Read the model definition and answer for the solid it produces. Units are mm, in the model's axes. A direction names the side the tool comes from. Round coordinates to 2 decimals unless told otherwise and drop trailing zeros. Order: outer loops, then holes, each group sorted by start corner. A loop starts at its lowest first (then second) coordinate and runs counter-clockwise, first axis right, second up. Notation, with made-up numbers: (46.25, 74) -> (74.25, 74) arc R10 cw to (74.25, 91) -> close; hole circle Ø11 at (-35.75, 83). An arc over 180 degrees is marked (long way). Use a Markdown table: item, result. Add a question column.
1. Section A-A, the plane z = 3.25 is taken. Give the vertices of the cut face in (x, y), then the cut area to 3 significant figures.
2. Section C-C, the plane x = 70 is taken. Give the vertices of the cut face in (y, z).
3. Given pin 1 (2.5 mm diameter, centred on y = -5.5, z = 18, fed in from +X); pin 2 (10 mm diameter, centred on x = 169.5, z = 6.5, fed in from -Y); pin 3 (4 mm diameter, centred on x = 310, z = 10, fed in from -Y); pin 4 (4.5 mm diameter, centred on x = 10, z = 10, fed in from +Y), each flat-ended and moving along its own axis, determine where each tip first touches the part or whether it passes through.
4. Consider L1, parallel to X at y = 13.95, z = 10; L2, parallel to Z at x = 10, y = 13.2; L3, parallel to X at y = 12, z = 12. Determine where each line is inside the solid, lowest interval first. Write a range as [from, to].
5. The mould has two halves that part along Y. Classify faces 1 (the face through (20, -12, 18)), 2 (the face through (10, -33, 18)), 3 (the face through (10, -12, 15)), 4 (the face through (158, 15, 10)): +Y half, -Y half, draft (parallel to the pull), parting line (faces both ways), or undercut.
6. Section B-B, the plane y = -15.8 is taken. Give the vertices of the cut face in (x, z), then the cut area to 4 significant figures.
7. Section D-D, the plane y = -28 is taken. Give the vertices of the cut face in (x, z), then the cut area to 3 significant figures.
8. For faces 5 (the face through (12.32, -17.93, 7.6)), 6 (the face through (9.46, 12.54, 12.44)), 7 (the face through (0, -4, 16)), determine the directions among +Z, -Z, +X, -X, +Y, -Y from which every point of the face is accessible in a straight line to the end or side of a thin tool.
Autodesk Inventor part; units mm, degrees
ref_plane "Plano de trabajo1" through (0, 10, 0) normal (0, 1, 0) x (1, 0, 0)
ref_plane "Plano de trabajo4" through (0, -3, 0) normal (0, -1, 0) x (1, 0, 0)
ref_plane "Plano de trabajo5" through (20, -33, 15) normal (0, 0, -1) x (-1, 0, 0)
ref_plane "Plano de trabajo1" through (0, 10, 0) normal (0, 1, 0) x (1, 0, 0)
sketch "Boceto3" plane through (0, 10, 0) normal (0, 1, 0) x (1, 0, 0)
  line L0 (20, -20) -> (0, -20)
  line L1 (0, 0) -> (20, 0)
  line L2 (0, -20) -> (20, -20)
  line L3 (20, -20) -> (20, 0)
  line L4 (20, 0) -> (0, 0)
  line L5 (0, 0) -> (0, -20)
extrude "Extrusión3" add sketch "Boceto3" along normal blind 5
ref_plane "Plano de trabajo4" through (0, -3, 0) normal (0, -1, 0) x (1, 0, 0)
sketch "Boceto8" plane through (0, -3, 0) normal (0, -1, 0) x (1, 0, 0)
  line L0 (0, 0) -> (0, 20)
  line L1 (0, 20) -> (20, 20)
  line L2 (0, 15) -> (20, 15)
  line L3 (20, 15) -> (20, 20)
  line L4 (20, 20) -> (0, 20)
  line L5 (0, 20) -> (0, 15)
  dimension "d25" = 5
extrude "Extrusión8" add sketch "Boceto8" along normal blind 30
ref_plane "Plano de trabajo5" through (20, -33, 15) normal (0, 0, -1) x (-1, 0, 0)
sketch "Boceto10" plane through (20, -33, 15) normal (0, 0, -1) x (-1, 0, 0)
  circle A0 centre (10, 17.2) radius 3.15
  line L0 (0, 33) -> (20, 33)
  line L1 (0, 32) -> (0, 0)
  point P0 (15.75, 33)
  point P1 (10, 33)
  dimension "d35" = 6.3
  dimension "d36" = 15.8
  dimension "d37" = 10
extrude "Extrusión9" add sketch "Boceto10" along normal blind 15
ref_plane "Plano de trabajo2" through (20, 10, 20) normal (1, 0, 0) x (0, 0, -1)
sketch "Boceto13" plane through (0, -3, 0) normal (0, 1, 0) x (1, 0, 0)
  line L0 (0, -20) -> (0, -15)
  line L1 (20, -15) -> (20, -20)
  line L2 (0, -15) -> (20, -15)
  line L3 (20, -15) -> (20, -20)
  line L4 (20, -20) -> (0, -20)
  line L5 (0, -20) -> (0, -15)
  point P0 (0, 0)
extrude "Extrusión12" add sketch "Boceto13" along normal blind 13
sketch "Boceto15" plane through (0, 15, 0) normal (0, 1, 0) x (1, 0, 0)
  circle A0 centre (10, -10) radius 2.5
  line L0 (0, 0) -> (0, -20)
  line L1 (0, -20) -> (20, -20)
  point P0 (320, -20)
  dimension "d58" = 5
  dimension "d59" = 10
  dimension "d60" = 10
extrude "Extrusión14" cut sketch "Boceto15" against normal blind 5
thread "Rosca6"
sketch "Boceto20" plane through (20, 10, 0) normal (1, 0, 0) x (0, 0, -1)
  line L0 (-20, 5) -> (0, 5)
  line L1 (-20, 5) -> (0, 5)
  line L2 (0, 5) -> (0, 0)
  line L3 (0, 0) -> (-20, 0)
  line L4 (-20, 0) -> (-20, 5)
  point P0 (0, -10)
extrude "Extrusión18" add sketch "Boceto20" along normal blind 300
sketch "Boceto21" plane through (0, 15, 0) normal (0, 1, 0) x (1, 0, 0)
  circle A0 centre (310, -10) radius 2.5
  line L0 (0, 0) -> (320, 0)
  line L1 (320, 0) -> (320, -20)
  dimension "d84" = 5
  dimension "d85" = 10
  dimension "d86" = 10
extrude "Extrusión19" cut sketch "Boceto21" against normal blind 300
thread "Rosca8"
properties part number "Ejes Base - C15_3DPrint"
Verdict:
| question | item | result |
|---|---|---|
| 1 | outline | (0, 10) -> (320, 10) -> (320, 15) -> (0, 15) -> close; circle Ø6.3 at (10, -15.8) |
| 1 | area | 1,630 mm2 |
| 2 | outline | (10, 0) -> (15, 0) -> (15, 20) -> (10, 20) -> close |
| 3 | pin 1 | stops at x = 20 |
| 3 | pin 2 | stops at y = 10 |
| 3 | pin 3 | passes through |
| 3 | pin 4 | stops at y = -12.65 |
| 4 | L1 | x = [0, 7.5], [12.5, 307.5], [312.5, 320] |
| 4 | L2 | z = [0, 7.5], [12.5, 20] |
| 4 | L3 | x = [0, 8.5], [11.5, 308.5], [311.5, 320] |
| 5 | face 1 | draft |
| 5 | face 2 | -Y half |
| 5 | face 3 | undercut |
| 5 | face 4 | +Y half |
| 6 | outline | (0, 15) -> (6.85, 15) -> (6.85, 0) -> (13.15, 0) -> (13.15, 15) -> (20, 15) -> (20, 20) -> (0, 20) -> close |
| 6 | area | 194.5 mm2 |
| 7 | outline | (0, 15) -> (20, 15) -> (20, 20) -> (0, 20) -> close |
| 7 | area | 100 mm2 |
| 8 | face 5 | -Z |
| 8 | face 6 | +Y |
| 8 | face 7 | +Z, -Z, -X, +Y, -Y |
